from build123d import *

# Parameters (mm, degrees)
SKETCH1_W           = 120
SKETCH1_H           = 70
SKETCH1_R           = 13.333333333
BOSS_EXTRUDE1_DEPTH = 14
BOSS_EXTRUDE2_DEPTH = 7.3
SKETCH4_R           = 21.666666667
CUT_EXTRUDE1_DEPTH  = 172.159351628
FILLET1_R           = 5
FILLET2_R           = 5
SCALE1_SCALE        = 0.15
FILLET3_START       = -4.2
FILLET3_DEPTH       = 1.095
FILLET3_START_2     = 3.105
FILLET3_2_DEPTH     = 1.095


with BuildPart() as part:
    # Sketch1 → Boss-Extrude1 (new body)
    with BuildSketch(Plane.XY):
        Rectangle(SKETCH1_W, SKETCH1_H)
        Circle(SKETCH1_R, mode=Mode.SUBTRACT)
    extrude(amount=BOSS_EXTRUDE1_DEPTH)

    # Sketch3 → Boss-Extrude2 (add)
    with BuildSketch(Plane(origin=(0, -28, 0), x_dir=(-1, 0, 0), z_dir=(0, -1, 0))):
        Polygon((55.436544165, -14), (-54.063561803, -14), (-16.446396869, -147.399198267), (17.819379231, -147.399198267), align=None)
    boss_extrude2 = extrude(amount=-BOSS_EXTRUDE2_DEPTH)

    # Mirror1: Boss-Extrude2 across plane
    add(boss_extrude2.mirror(Plane.ZX))

    # Sketch4 → Cut-Extrude1 (cut, through all)
    with BuildSketch(Plane.XZ.offset(28)):
        with Locations(Location((-0.686491181, 90.853024988, 0), (0, 0, 90))):
            Circle(SKETCH4_R)
    extrude(amount=-CUT_EXTRUDE1_DEPTH, mode=Mode.SUBTRACT)

    # Fillet1
    # the kernel refuses this fillet: 5 mm, written as the material it takes off along each edge
    with BuildSketch(Plane(origin=(-55, 30, 9), x_dir=(0, 0, 1), z_dir=(-1, 0, 0))) as fillet1_piece_1_section:
        Polygon((0, 0), (FILLET1_R * 1.02, 0), (FILLET1_R * 1.02, FILLET1_R * 1.02), (0, FILLET1_R * 1.02), align=None)
    fillet1_piece_1 = extrude(amount=FILLET1_R * 1.02, mode=Mode.PRIVATE)
    fillet1_piece_1 = fillet1_piece_1 - Plane(origin=(-55, 30, 9), x_dir=(0, -0.7071067811865475, -0.7071067811865475), z_dir=(-1, 0, 0)) * Sphere(FILLET1_R, mode=Mode.PRIVATE)
    add(fillet1_piece_1, mode=Mode.SUBTRACT)
    with BuildSketch(Plane(origin=(-55, -30, 9), x_dir=(-1, 0, 0), z_dir=(0, -1, 0))) as fillet1_piece_2_section:
        Polygon((0, 0), (FILLET1_R * 1.02, 0), (FILLET1_R * 1.02, -FILLET1_R * 1.02), (0, -FILLET1_R * 1.02), align=None)
    fillet1_piece_2 = extrude(amount=FILLET1_R * 1.02, mode=Mode.PRIVATE)
    fillet1_piece_2 = fillet1_piece_2 - Plane(origin=(-55, -30, 9), x_dir=(0.7071067811865475, 0, -0.7071067811865475), z_dir=(0, -1, 0)) * Sphere(FILLET1_R, mode=Mode.PRIVATE)
    add(fillet1_piece_2, mode=Mode.SUBTRACT)
    with BuildSketch(Plane(origin=(-55, 30, 5), x_dir=(0, 0, -1), z_dir=(-1, 0, 0))) as fillet1_piece_3_section:
        Polygon((0, 0), (FILLET1_R * 1.02, 0), (FILLET1_R * 1.02, -FILLET1_R * 1.02), (0, -FILLET1_R * 1.02), align=None)
    fillet1_piece_3 = extrude(amount=FILLET1_R * 1.02, mode=Mode.PRIVATE)
    fillet1_piece_3 = fillet1_piece_3 - Plane(origin=(-55, 30, 5), x_dir=(0, -0.7071067811865475, 0.7071067811865475), z_dir=(-1, 0, 0)) * Sphere(FILLET1_R, mode=Mode.PRIVATE)
    add(fillet1_piece_3, mode=Mode.SUBTRACT)
    with BuildSketch(Plane(origin=(-55, -30, 5), x_dir=(-1, 0, 0), z_dir=(0, -1, 0))) as fillet1_piece_4_section:
        Polygon((0, 0), (FILLET1_R * 1.02, 0), (FILLET1_R * 1.02, FILLET1_R * 1.02), (0, FILLET1_R * 1.02), align=None)
    fillet1_piece_4 = extrude(amount=FILLET1_R * 1.02, mode=Mode.PRIVATE)
    fillet1_piece_4 = fillet1_piece_4 - Plane(origin=(-55, -30, 5), x_dir=(0.7071067811865475, 0, 0.7071067811865475), z_dir=(0, -1, 0)) * Sphere(FILLET1_R, mode=Mode.PRIVATE)
    add(fillet1_piece_4, mode=Mode.SUBTRACT)
    with BuildSketch(Plane(origin=(55, 30, 9), x_dir=(0, 0, 1), z_dir=(1, 0, 0))) as fillet1_piece_5_section:
        Polygon((0, 0), (FILLET1_R * 1.02, 0), (FILLET1_R * 1.02, -FILLET1_R * 1.02), (0, -FILLET1_R * 1.02), align=None)
    fillet1_piece_5 = extrude(amount=FILLET1_R * 1.02, mode=Mode.PRIVATE)
    fillet1_piece_5 = fillet1_piece_5 - Plane(origin=(55, 30, 9), x_dir=(0, -0.7071067811865475, -0.7071067811865475), z_dir=(1, 0, 0)) * Sphere(FILLET1_R, mode=Mode.PRIVATE)
    add(fillet1_piece_5, mode=Mode.SUBTRACT)
    with BuildSketch(Plane(origin=(55, 30, 5), x_dir=(0, 0, -1), z_dir=(1, 0, 0))) as fillet1_piece_6_section:
        Polygon((0, 0), (FILLET1_R * 1.02, 0), (FILLET1_R * 1.02, FILLET1_R * 1.02), (0, FILLET1_R * 1.02), align=None)
    fillet1_piece_6 = extrude(amount=FILLET1_R * 1.02, mode=Mode.PRIVATE)
    fillet1_piece_6 = fillet1_piece_6 - Plane(origin=(55, 30, 5), x_dir=(0, -0.7071067811865475, 0.7071067811865475), z_dir=(1, 0, 0)) * Sphere(FILLET1_R, mode=Mode.PRIVATE)
    add(fillet1_piece_6, mode=Mode.SUBTRACT)
    with BuildSketch(Plane(origin=(55, -30, 9), x_dir=(1, 0, 0), z_dir=(0, -1, 0))) as fillet1_piece_7_section:
        Polygon((0, 0), (FILLET1_R * 1.02, 0), (FILLET1_R * 1.02, FILLET1_R * 1.02), (0, FILLET1_R * 1.02), align=None)
    fillet1_piece_7 = extrude(amount=FILLET1_R * 1.02, mode=Mode.PRIVATE)
    fillet1_piece_7 = fillet1_piece_7 - Plane(origin=(55, -30, 9), x_dir=(-0.7071067811865475, 0, -0.7071067811865475), z_dir=(0, -1, 0)) * Sphere(FILLET1_R, mode=Mode.PRIVATE)
    add(fillet1_piece_7, mode=Mode.SUBTRACT)
    with BuildSketch(Plane(origin=(55, -30, 5), x_dir=(1, 0, 0), z_dir=(0, -1, 0))) as fillet1_piece_8_section:
        Polygon((0, 0), (FILLET1_R * 1.02, 0), (FILLET1_R * 1.02, -FILLET1_R * 1.02), (0, -FILLET1_R * 1.02), align=None)
    fillet1_piece_8 = extrude(amount=FILLET1_R * 1.02, mode=Mode.PRIVATE)
    fillet1_piece_8 = fillet1_piece_8 - Plane(origin=(55, -30, 5), x_dir=(-0.7071067811865475, 0, 0.7071067811865475), z_dir=(0, -1, 0)) * Sphere(FILLET1_R, mode=Mode.PRIVATE)
    add(fillet1_piece_8, mode=Mode.SUBTRACT)
    with BuildSketch(Plane(origin=(-60, 30, 14), x_dir=(0, 0, -1), z_dir=(0, -1, 0))) as fillet1_piece_9_section:
        with BuildLine():
            CenterArc((FILLET1_R, FILLET1_R), FILLET1_R, 180, 90)
            Line((0, FILLET1_R), (0, 0))
            Line((0, 0), (FILLET1_R, 0))
        make_face()
    fillet1_piece_9 = extrude(amount=60, mode=Mode.PRIVATE)
    fillet1_piece_9 = split(fillet1_piece_9, bisect_by=Plane(origin=(-55.772691467, 30, 12.807943643), z_dir=(-0.9624652257513497, 0, 0.2714050279921198)), keep=Keep.TOP, mode=Mode.PRIVATE)
    add(fillet1_piece_9, mode=Mode.SUBTRACT)
    with BuildSketch(Plane(origin=(-60, 30, 14), x_dir=(0, 0, -1), z_dir=(0, -1, 0))) as fillet1_piece_10_section:
        with BuildLine():
            CenterArc((FILLET1_R, FILLET1_R), FILLET1_R, 180, 90)
            Line((0, FILLET1_R), (0, 0))
            Line((0, 0), (FILLET1_R, 0))
        make_face()
    fillet1_piece_10 = extrude(amount=60, mode=Mode.PRIVATE)
    fillet1_piece_10 = split(fillet1_piece_10, bisect_by=Plane(origin=(-60, 28, 14), z_dir=(0, 1, 0)), keep=Keep.TOP, mode=Mode.PRIVATE)
    add(fillet1_piece_10, mode=Mode.SUBTRACT)
    with BuildSketch(Plane(origin=(-60, 30, 14), x_dir=(0, 0, -1), z_dir=(0, -1, 0))) as fillet1_piece_11_section:
        with BuildLine():
            CenterArc((FILLET1_R, FILLET1_R), FILLET1_R, 180, 90)
            Line((0, FILLET1_R), (0, 0))
            Line((0, 0), (FILLET1_R, 0))
        make_face()
    fillet1_piece_11 = extrude(amount=60, mode=Mode.PRIVATE)
    fillet1_piece_11 = split(fillet1_piece_11, bisect_by=Plane(origin=(-60, -20.7, 14), z_dir=(0, 1, 0)), keep=Keep.TOP, mode=Mode.PRIVATE)
    fillet1_piece_11 = split(fillet1_piece_11, bisect_by=Plane(origin=(-60, 20.7, 14), z_dir=(0, -1, 0)), keep=Keep.TOP, mode=Mode.PRIVATE)
    add(fillet1_piece_11, mode=Mode.SUBTRACT)
    with BuildSketch(Plane(origin=(-60, 30, 14), x_dir=(0, 0, -1), z_dir=(0, -1, 0))) as fillet1_piece_12_section:
        with BuildLine():
            CenterArc((FILLET1_R, FILLET1_R), FILLET1_R, 180, 90)
            Line((0, FILLET1_R), (0, 0))
            Line((0, 0), (FILLET1_R, 0))
        make_face()
    fillet1_piece_12 = extrude(amount=60, mode=Mode.PRIVATE)
    fillet1_piece_12 = split(fillet1_piece_12, bisect_by=Plane(origin=(-60, -28, 14), z_dir=(0, -1, 0)), keep=Keep.TOP, mode=Mode.PRIVATE)
    add(fillet1_piece_12, mode=Mode.SUBTRACT)
    with BuildSketch(Plane(origin=(-60, 30, 0), x_dir=(0, 0, 1), z_dir=(0, -1, 0)), Plane(origin=(60, -30, 0), x_dir=(0, 0, 1), z_dir=(0, 1, 0))) as fillet1_piece_13:
        with BuildLine():
            CenterArc((FILLET1_R, -FILLET1_R), FILLET1_R, 90, 90)
            Line((0, -FILLET1_R), (0, 0))
            Line((0, 0), (FILLET1_R, 0))
        make_face()
    extrude(amount=60, mode=Mode.SUBTRACT)
    with BuildSketch(Plane(origin=(55, 35, 14), x_dir=(0, -1, 0), z_dir=(-1, 0, 0)), Plane(origin=(-55, -35, 0), x_dir=(0, 0, 1), z_dir=(1, 0, 0))) as fillet1_piece_14:
        with BuildLine():
            CenterArc((FILLET1_R, -FILLET1_R), FILLET1_R, 90, 90)
            Line((0, -FILLET1_R), (0, 0))
            Line((0, 0), (FILLET1_R, 0))
        make_face()
    extrude(amount=110, mode=Mode.SUBTRACT)
    with BuildSketch(Plane(origin=(-60, 35, 5), x_dir=(0, -1, 0), z_dir=(0, 0, 1)), Plane(origin=(-60, -35, 5), x_dir=(1, 0, 0), z_dir=(0, 0, 1))) as fillet1_piece_15:
        with BuildLine():
            CenterArc((FILLET1_R, FILLET1_R), FILLET1_R, 180, 90)
            Line((0, FILLET1_R), (0, 0))
            Line((0, 0), (FILLET1_R, 0))
        make_face()
    extrude(amount=4, mode=Mode.SUBTRACT)
    with BuildSketch(Plane(origin=(55, 35, 0), x_dir=(0, -1, 0), z_dir=(-1, 0, 0)), Plane(origin=(-55, -35, 14), x_dir=(0, 0, -1), z_dir=(1, 0, 0))) as fillet1_piece_16:
        with BuildLine():
            CenterArc((FILLET1_R, FILLET1_R), FILLET1_R, 180, 90)
            Line((0, FILLET1_R), (0, 0))
            Line((0, 0), (FILLET1_R, 0))
        make_face()
    extrude(amount=110, mode=Mode.SUBTRACT)
    with BuildSketch(Plane(origin=(60, -30, 14), x_dir=(0, 0, -1), z_dir=(0, 1, 0))) as fillet1_piece_17:
        with BuildLine():
            CenterArc((FILLET1_R, FILLET1_R), FILLET1_R, 180, 90)
            Line((0, FILLET1_R), (0, 0))
            Line((0, 0), (FILLET1_R, 0))
        make_face()
    extrude(amount=60, mode=Mode.SUBTRACT)
    with BuildSketch(Plane(origin=(60, 35, 5), x_dir=(0, -1, 0), z_dir=(0, 0, 1)), Plane(origin=(60, -35, 5), x_dir=(-1, 0, 0), z_dir=(0, 0, 1))) as fillet1_piece_18:
        with BuildLine():
            CenterArc((FILLET1_R, -FILLET1_R), FILLET1_R, 90, 90)
            Line((0, -FILLET1_R), (0, 0))
            Line((0, 0), (FILLET1_R, 0))
        make_face()
    extrude(amount=4, mode=Mode.SUBTRACT)

    # Fillet2
    fillet2_edges = [part.edges().sort_by_distance(p)[0] for p in [
        (-17.819379231, -24.35, 147.399198267),
        (16.446396869, -24.35, 147.399198267),
        (16.446396869, 24.35, 147.399198267),
        (-17.819379231, 24.35, 147.399198267),
    ]]
    fillet(fillet2_edges, radius=FILLET2_R)


with BuildPart() as part_1:
    # Scale1: scaled about (-0.362902499, 0, 37.686238577)
    add(part.part.scale(SCALE1_SCALE).moved(Location((-0.308467124, 0, 32.03330279))))

    # Fillet3: read off the stored shape, not the designer's step
    # Fillet3 outline → Fillet3 (add)
    with BuildSketch(Plane(origin=(0, 0, 0), x_dir=(1, 0, 0), z_dir=(0, 1, 0)).offset(FILLET3_START)):
        with BuildLine():
            ThreePointArc((-8.624776975, -34.130365708), (-8.945174574, -34.025920365), (-9.187499582, -33.791736588))
            ThreePointArc((-9.187499582, -33.791736588), (-8.465735644, -35.11094716), (-7.949946764, -36.523470273))
            Line((-7.949946764, -36.523470273), (-8.624776975, -34.130365708))
        make_face()
        with BuildLine():
            Line((7.941532876, -34.13330279), (7.801067146, -34.13330279))
            Line((7.801067146, -34.13330279), (6.984932745, -37.027504812))
            ThreePointArc((6.984932745, -37.027504812), (7.621987061, -35.357141421), (8.546280698, -33.826901788))
            ThreePointArc((8.546280698, -33.826901788), (8.280502455, -34.052331656), (7.941532876, -34.13330279))
        make_face()
    extrude(amount=FILLET3_DEPTH)

    # Fillet3 2 outline → Fillet3 2 (add)
    with BuildSketch(Plane(origin=(0, 0, 0), x_dir=(1, 0, 0), z_dir=(0, 1, 0)).offset(FILLET3_START_2)):
        with BuildLine():
            ThreePointArc((-8.624776975, -34.130365708), (-8.945174574, -34.025920365), (-9.187499582, -33.791736588))
            ThreePointArc((-9.187499582, -33.791736588), (-8.465735644, -35.11094716), (-7.949946764, -36.523470273))
            Line((-7.949946764, -36.523470273), (-8.624776975, -34.130365708))
        make_face()
        with BuildLine():
            Line((7.941532876, -34.13330279), (7.801067146, -34.13330279))
            Line((7.801067146, -34.13330279), (6.984932745, -37.027504812))
            ThreePointArc((6.984932745, -37.027504812), (7.621987061, -35.357141421), (8.546280698, -33.826901788))
            ThreePointArc((8.546280698, -33.826901788), (8.280502455, -34.052331656), (7.941532876, -34.13330279))
        make_face()
    extrude(amount=FILLET3_2_DEPTH)


solid = part_1.part
Could you check a few things on this model? Use its own coordinates, in mm. A direction names the side the tool comes from. Coordinates: 2 decimals unless noted, no trailing zeros. Loops run counter-clockwise (first coordinate to the right, second up) from the corner with the lowest first, then second, coordinate; pieces in that order, holes last.
1. I need wall thicknesses on L1, parallel to Y at x = -6.75, z = 36 (3 decimals); L2, parallel to Z at x = 1.5, y = -1; L3, parallel to Z at x = -1, y = -4 (3 decimals). Which ranges of each line are inside material? Lowest first, please.
2. Imagine slicing it at B-B (z = 46.5). Please give me the cut outline in (x, y) (3 decimals).
3. We'd pull the mould along Y, two halves only. Please class faces 1 (the face through (-5.51, 3.66, 45.18)), 2 (the face through (0, -3.105, 42)), 3 (the face through (0, 4.2, 42)): released by +Y, released by -Y, zero draft, split by the parting line, or undercut.
4. For P1, Ø4, axis at y = 3, z = 44.5, coming from the -X side; P2, Ø9, axis at x = 0, z = 46, coming from the +Y side; P3, Ø5, axis at y = 3, z = 45.5, coming from the -X side, each with a flat end and sliding along its axis, tell me the tip position at first contact or that it passes through.
5. Imagine slicing it at D-D (y = 1.5). Please give me the cut outline in (x, z), and give its area (3 significant figures).
6. Imagine slicing it at C-C (x = 1). Please give me the cut outline in (y, z) (3 decimals), and give its area (3 significant figures).
7. For faces 4 (the face through (-2.3, -1.3, 34.133)), 5 (the face through (-0.554, 3.645, 42.414)), which set-ups out of +Z, -Z, +X, -X, +Y, -Y let a thin tool reach every point of the face, with its end or its side?
8. Imagine slicing it at A-A (y = 0). Please give me the cut outline in (x, z).
Computed values:
1. L1: y = -4.2 to -3.105, 3.105 to 4.2
1. L2: z = 32.03 to 34.13
1. L3: z = 32.033 to 42.465, 48.858 to 54.143
2. outline: (-5.137, -4.2) - (-3.551, -4.2) - (-3.551, -3.105) - (-5.137, -3.105) - close; (-5.137, 3.105) - (-3.551, 3.105) - (-3.551, 4.2) - (-5.137, 4.2) - close; (2.728, -4.2) - (4.314, -4.2) - (4.314, -3.105) - (2.728, -3.105) - close; (2.728, 3.105) - (4.314, 3.105) - (4.314, 4.2) - (2.728, 4.2) - close
3. face 1: zero draft
3. face 2: undercut
3. face 3: released by +Y
4. P1: stops at x = -6.26
4. P2: stops at y = 4.2
4. P3: stops at x = -6.12
5. outline: (-9.31, 32.78) arc R0.75 ccw to (-8.56, 32.03) - (-1.63, 32.03) - (-1.63, 34.13) - (-8.56, 34.13) arc R0.75 ccw to (-9.31, 33.38) - close; (1.01, 32.03) - (7.94, 32.03) arc R0.75 ccw to (8.69, 32.78) - (8.69, 33.38) arc R0.75 ccw to (7.94, 34.13) - (1.01, 34.13) - close
5. area: 31.8 mm2
6. outline: (-5.25, 32.783) arc R0.75 ccw to (-4.5, 32.033) - (-1.513, 32.033) - (-1.513, 34.133) - (-3.105, 34.133) - (-3.105, 42.734) - (-4.2, 42.734) - (-4.2, 34.133) - (-4.5, 34.133) arc R0.75 ccw to (-5.25, 33.383) - close; (-4.2, 48.589) - (-3.105, 48.589) - (-3.105, 54.143) - (-4.2, 54.143) - close; (1.513, 32.033) - (4.5, 32.033) arc R0.75 ccw to (5.25, 32.783) - (5.25, 33.383) arc R0.75 ccw to (4.5, 34.133) - (4.2, 34.133) - (4.2, 42.734) - (3.105, 42.734) - (3.105, 34.133) - (1.513, 34.133) - close; (3.105, 48.589) - (4.2, 48.589) - (4.2, 54.143) - (3.105, 54.143) - close
6. area: 46.2 mm2
7. face 4: +Z, +X, -X
7. face 5: +Y, -Y
8. outline: (-9.31, 32.78) arc R0.75 ccw to (-8.56, 32.03) - (-2.31, 32.03) - (-2.31, 34.13) - (-8.56, 34.13) arc R0.75 ccw to (-9.31, 33.38) - close; (1.69, 32.03) - (7.94, 32.03) arc R0.75 ccw to (8.69, 32.78) - (8.69, 33.38) arc R0.75 ccw to (7.94, 34.13) - (1.69, 34.13) - close
